from build123d import *

# Parameters (mm, degrees)
SKETCH1_W           = 22.225
SKETCH1_H           = 28.575
BOSS_EXTRUDE1_DEPTH = 3.175
FILLET1_R           = 6.35
SKETCH2_R           = 3.175
CUT_EXTRUDE1_DEPTH  = 19.376641083


with BuildPart() as part:
    # Sketch1 → Boss-Extrude1 (new body)
    with BuildSketch(Plane.XY):
        Rectangle(SKETCH1_W, SKETCH1_H)
    extrude(amount=BOSS_EXTRUDE1_DEPTH)

    # Fillet1
    fillet1_edges = [part.edges().sort_by_distance(p)[0] for p in [
        (-11.1125, 14.2875, 1.5875),
        (11.1125, 14.2875, 1.5875),
    ]]
    fillet(fillet1_edges, radius=FILLET1_R)

    # Sketch2 → Cut-Extrude1 (cut, through all)
    with BuildSketch(Plane.XY.offset(3.175)):
        with Locations((0, 4.7625)):
            Circle(SKETCH2_R)
    extrude(amount=-CUT_EXTRUDE1_DEPTH, mode=Mode.SUBTRACT)


solid = part.part
Model file for the job. Use its own axes, mm. Coordinates: 2 decimals unless noted, no trailing zeros. Write each loop counter-clockwise with the first axis right and the second up, starting at its lowest first coordinate (ties: lowest second). Pieces come first, ordered by that corner, then holes. Notation, with made-up numbers: (53, -26) - (80, -26) arc R16 cw to (80, -6) - close; hole circle Ø2 at (42, 48.5). An arc over 180 degrees is marked (long way). Write each question's results on one line, items separated by ' | '. Start each with the question number.
1) Mould opens along Y. For faces 1 (the face through (0, -14.288, 2)), 2 (the face through (0, 14.288, 2)), 3 (the face through (-0.688, 1.663, 1.61)), 4 (the face through (11.112, -3, 2)) say: pulls with the +Y half, pulls with the -Y half, needs draft (parallel to the pull), parting line crosses it, or undercut.
2) Cut at B-B (x = 0). Write the cut outline in (y, z) (1 decimal), then the cut area to 3 significant figures.
3) Probe line 1 along Y through (x, z) = (0, 2.05); line 2 along X through (y, z) = (2.25, 1.1); line 3 along X through (y, z) = (4, 2.45). List the from-to ranges inside material, lowest first. Write a range as from..to.
4) Cut at C-C (x = 8). Write the cut outline in (y, z) (1 decimal).
Returned:
1) face 1: pulls with the -Y half | face 2: pulls with the +Y half | face 3: undercut | face 4: needs draft
2) outline: (-14.3, 0) - (1.6, 0) - (1.6, 3.2) - (-14.3, 3.2) - close; (7.9, 0) - (14.3, 0) - (14.3, 3.2) - (7.9, 3.2) - close | area: 70.6 mm^2
3) line 1: -14.29..1.59, 7.94..14.29 | line 2: -11.11..-1.94, 1.94..11.11 | line 3: -11.11..-3.08, 3.08..11.11
4) outline: (-14.3, 0) - (13.4, 0) - (13.4, 3.2) - (-14.3, 3.2) - close
